from build123d import *

# Parameters (mm, degrees)
F1_DEPTH = 5.08


with BuildPart() as f1:
    # F0 (on Top) → F1 (new body)
    with BuildSketch(Plane.XY):
        with BuildLine():
            ThreePointArc((-52.720005, -30.842755), (-41.509299, -56.359582), (-63.5, -73.48259))
            Line((-63.5, -73.48259), (-63.5, -101.6))
            ThreePointArc((-63.5, -101.6), (-47.625, -85.725), (-31.75, -101.6))
            ThreePointArc((-31.75, -101.6), (-15.875, -85.725), (0, -101.6))
            Line((0, -101.6), (0, -73.48259))
            ThreePointArc((0, -73.48259), (-22.056218, -56.093689), (-10.29501, -30.588304))
            ThreePointArc((-10.29501, -30.588304), (-6.878118, -25.733334), (-8.967166, -20.176198))
            Line((-8.967166, -20.176198), (-27.540063, -3.728268))
            ThreePointArc((-27.540063, -3.728268), (-31.75, -2.132102), (-35.959937, -3.728268))
            Line((-35.959937, -3.728268), (-54.003646, -19.707556))
            ThreePointArc((-54.003646, -19.707556), (-56.263112, -25.609609), (-52.720005, -30.842755))
        make_face()
    extrude(amount=F1_DEPTH)


solid = f1.part
Design review of the part built by this model. Coordinates are the model's own, in mm. Give positions to 0.01 mm unless a question says otherwise; leave off trailing zeros. Order: outer loops, then holes, each group sorted by start corner. A loop starts at its lowest first (then second) coordinate and runs counter-clockwise, first axis right, second up.
1. Add section C-C, the plane y = -92. State the section outline as (x, z) points, then the cut area to 3 significant figures.
Solution:
outline: (-63.5, 0) - (-60.27, 0) - (-60.27, 5.08) - (-63.5, 5.08) - close; (-34.98, 0) - (-28.52, 0) - (-28.52, 5.08) - (-34.98, 5.08) - close; (-3.23, 0) - (0, 0) - (0, 5.08) - (-3.23, 5.08) - close
area: 65.7 mm2
2. Add section B-B, the plane x = -21. State the section outline as (y, z) points.
Solution:
outline: (-86.58, 0) - (-59.37, 0) - (-59.37, 5.08) - (-86.58, 5.08) - close; (-42.23, 0) - (-9.52, 0) - (-9.52, 5.08) - (-42.23, 5.08) - close
3. Add section A-A, the plane z = 1.35. State the section outline as (x, y) points (3 decimals).
Solution:
outline: (-63.5, -101.6) arc R15.875 cw to (-31.75, -101.6) arc R15.875 cw to (0, -101.6) - (0, -73.483) arc R22.683 cw to (-10.295, -30.588) arc R6.35 ccw to (-8.967, -20.176) - (-27.54, -3.728) arc R6.35 ccw to (-35.96, -3.728) - (-54.004, -19.708) arc R6.838 ccw to (-52.72, -30.843) arc R22.683 cw to (-63.5, -73.483) - close
4. For pin 1 Ø1.5 at (x, z) = (-17, 4) entering from -Y, flat-tipped, find the tip position at first contact; note if it passes through.
Solution:
pin 1: stops at y = -85.84
5. Mouldability with a two-part tool opening along Y and no side actions: class faces 1 (the cylindrical face through (-31.686, -2.132, 2.504)), 2 (the cylindrical face through (-16.22, -85.73, 2.5)), 3 (the cylindrical face through (-6.89, -25.82, 2.5)) as +Y half, -Y half, draft (parallel to the pull), parting line (faces both ways), or undercut.
Solution:
face 1: +Y half
face 2: -Y half
face 3: undercut
6. To check wall thickness, follow L1, parallel to X at y = -87.5, z = 0.45; L2, parallel to X at y = -92, z = 4.45; L3, parallel to Y at x = -9, z = 2.9. State the ranges of each line that lie inside material, in increasing order.
Solution:
L1: x = -63.5 to -54.92, -40.33 to -23.17, -8.58 to 0
L2: x = -63.5 to -60.27, -34.98 to -28.52, -3.23 to 0
L3: y = -87.29 to -71.62, -29.71 to -20.15
7. Add section D-D, the plane y = -11.5. State the section outline as (x, z) points.
Solution:
outline: (-44.74, 0) - (-18.76, 0) - (-18.76, 5.08) - (-44.74, 5.08) - close
